from build123d import *

# Parameters (mm, degrees)
F0_W     = 31.75
F0_H     = 19.05
F0_R     = 6
F1_DEPTH = 4.7625
F3_D     = 2.9464


with BuildPart() as f1:
    # F0 (on Front) → F1 (new body, symmetric)
    with BuildSketch(Plane.XZ):
        Rectangle(F0_W, F0_H)
        Circle(F0_R, mode=Mode.SUBTRACT)
    extrude(amount=F1_DEPTH, both=True)

    # F3 (through all)
    with Locations(Plane.XY.offset(9.525)):
        with Locations((-11.1125, 0), (11.1125, 0)):
            Hole(F3_D / 2)


solid = f1.part
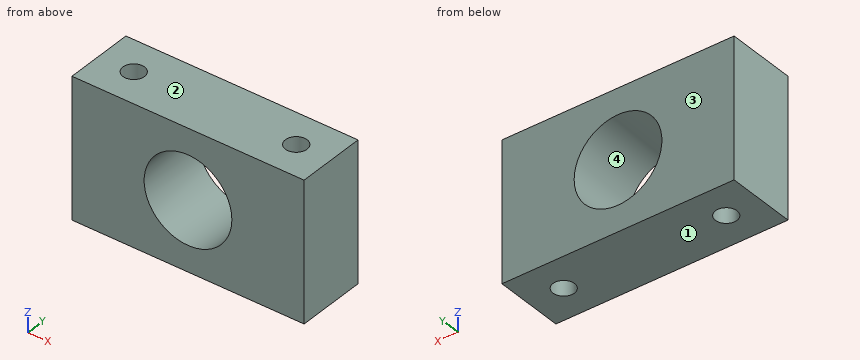
Verification items for the finished model (mm, model axes). Face numbers are marked on the shaded views. Coordinates: 2 decimals unless noted, no trailing zeros. Write each loop counter-clockwise with the first axis right and the second up, starting at its lowest first coordinate (ties: lowest second). Pieces come first, ordered by that corner, then holes. Notation, with made-up numbers: (34.5, -32) - (58.5, -32) arc R24 ccw to (58.5, 0) - close; hole circle Ø3 at (33, 69). An arc over 180 degrees is marked (long way). Answer as a JSON object with one key per item and string values.
(1) Mould release check, pull along Z, two halves, no side actions. Record for the marked faces 1, 2, 3 and 4: pulls with the +Z half, pulls with the -Z half, needs draft (parallel to the pull), parting line crosses it, or undercut.
Report:
{"face 1": "pulls with the -Z half", "face 2": "pulls with the +Z half", "face 3": "needs draft", "face 4": "undercut"}
(2) Cross-section at A-A on y = 0. Record the cut outline in (x, z) (3 decimals), plus the area to 3 significant figures.
Report:
{"outline": "(-15.875, -9.525) - (-12.586, -9.525) - (-12.586, 9.525) - (-15.875, 9.525) - close; (-9.639, -9.525) - (9.639, -9.525) - (9.639, 9.525) - (-9.639, 9.525) - close; (12.586, -9.525) - (15.875, -9.525) - (15.875, 9.525) - (12.586, 9.525) - close; hole circle Ø12 at (0, 0)", "area": "379 mm^2"}
(3) Cross-section at D-D on z = -7.75. Record the cut outline in (x, y) (1 decimal).
Report:
{"outline": "(-15.9, -4.8) - (15.9, -4.8) - (15.9, 4.8) - (-15.9, 4.8) - close; hole circle Ø2.9 at (-11.1, 0); hole circle Ø2.9 at (11.1, 0)"}
(4) Cross-section at B-B on z = 0. Record the cut outline in (x, y) (1 decimal).
Report:
{"outline": "(-15.9, -4.8) - (-6, -4.8) - (-6, 4.8) - (-15.9, 4.8) - close; (6, -4.8) - (15.9, -4.8) - (15.9, 4.8) - (6, 4.8) - close; hole circle Ø2.9 at (-11.1, 0); hole circle Ø2.9 at (11.1, 0)"}
(5) Thickness scan on line 1 along Y through (x, z) = (11, -6.75); line 2 along Z through (x, y) = (0, -0.25) (3 decimals); line 3 along X through (y, z) = (1.25, -1.75) (3 decimals). Record the ranges inside material, lowest first.
Report:
{"line 1": "-4.76 to -1.47, 1.47 to 4.76", "line 2": "-9.525 to -6, 6 to 9.525", "line 3": "-15.875 to -11.892, -10.333 to -5.739, 5.739 to 10.333, 11.892 to 15.875"}
(6) Cross-section at C-C on x = 0. Record the cut outline in (y, z) (1 decimal), plus the area to 3 significant figures.
Report:
{"outline": "(-4.8, -9.5) - (4.8, -9.5) - (4.8, -6) - (-4.8, -6) - close; (-4.8, 6) - (4.8, 6) - (4.8, 9.5) - (-4.8, 9.5) - close", "area": "67.2 mm^2"}
